Here's how the part is built. I have some questions about the finished solid (model axes, mm). A direction names the side the tool comes from. Coordinates: 2 decimals unless noted, no trailing zeros. Write each loop counter-clockwise with the first axis right and the second up, starting at its lowest first coordinate (ties: lowest second). Pieces come first, ordered by that corner, then holes.
(1) Which directions (+Z, -Z, +X, -X, +Y, -Y) give clear straight access to the entire face, cutting with the end or side of a thin tool? Please do faces 4 (the flat face through (-1, 106, 50)), 5 (the flat face through (-1, 85, 53)), 6 (the flat face through (-1, 86, -55)).
(2) Please list where these lines run through material, in increasing order: probe 1 along X at (y, z) = (111, 12); probe 2 along Z at (x, y) = (2, 154); probe 3 along Y at (x, z) = (-9, -48).
(3) Imagine slicing it at C-C, the plane z = -33.5. List the corners of the cut face in (x, y) for me, plus the area to 4 significant figures.
(4) For pin 1 Ø8 at (x, y) = (-37.5, 79) entering from +Z, with a flat end and sliding along its axis, tell me the tip position at first contact or that it passes through.
(5) Thinking about a two-plate mould opening in Y: for faces 1 (the flat face through (-1, 5, 53)), 2 (the flat face through (-1, 86, -50)), 3 (the flat face through (-1, 0, 1)), which applies, released by +Y, released by -Y, zero draft, split by the parting line, or undercut?
(6) Imagine slicing it at B-B, the plane y = 93. List the corners of the cut face in (x, z) for me.
(7) Imagine slicing it at A-A, the plane x = -57. List the corners of the cut face in (y, z) for me.
```python
from build123d import *

# Parameters (mm, degrees)
SKETCH1_W           = 185
SKETCH1_H           = 110
SKETCH1_W_2         = 175
SKETCH1_H_2         = 100
EXTRUDE_THIN1_DEPTH = 175
SKETCH2_W           = 185
SKETCH2_H           = 110
BOSS_EXTRUDE2_DEPTH = 5
CUT_EXTRUDE2_REACH  = 228.454
SKETCH5_W           = 130
SKETCH5_H           = 80
SKETCH6_R           = 1.5
BOSS_EXTRUDE3_DEPTH = 2


with BuildPart() as part:
    # Sketch1 → Extrude-Thin1 (new body)
    with BuildSketch(Plane(origin=(0, 0, 0), x_dir=(1, 0, 0), z_dir=(0, 1, 0))):
        Rectangle(SKETCH1_W, SKETCH1_H)
        Rectangle(SKETCH1_W_2, SKETCH1_H_2, mode=Mode.SUBTRACT)
    extrude(amount=EXTRUDE_THIN1_DEPTH)

    # Sketch2 → Boss-Extrude2 (add)
    with BuildSketch(Plane.XZ):
        Rectangle(SKETCH2_W, SKETCH2_H)
    extrude(amount=BOSS_EXTRUDE2_DEPTH)

    # Sketch5 → Cut-Extrude2 (cut, up to next)
    with BuildSketch(Plane.XY.offset(55), mode=Mode.PRIVATE) as cut_extrude2_sk1:
        with Locations((0, 45)):
            Rectangle(SKETCH5_W, SKETCH5_H)
    cut_extrude2_tool1 = extrude(cut_extrude2_sk1.sketch, amount=-CUT_EXTRUDE2_REACH, mode=Mode.PRIVATE) & part.part
    add(cut_extrude2_tool1.solids().sort_by_distance((0, 45, 55))[0], mode=Mode.SUBTRACT)

    # Sketch6 → Boss-Extrude3 (add)
    with BuildSketch(Plane.ZY.offset(-65)):
        with Locations(Location((52.5, 7.5, 0), (0, 0, 270))):
            Circle(SKETCH6_R)
    extrude(amount=BOSS_EXTRUDE3_DEPTH)


solid = part.part
```
Recorded:
1. face 4: +Y
1. face 5: +Z
1. face 6: -Z, +X, -X, +Y, -Y
2. probe 1: x = -92.5 to -87.5, 87.5 to 92.5
2. probe 2: z = -55 to -50, 50 to 55
2. probe 3: y = -5 to 0
3. outline: (-92.5, -5) - (92.5, -5) - (92.5, 175) - (87.5, 175) - (87.5, 0) - (-87.5, 0) - (-87.5, 175) - (-92.5, 175) - close
3. area: 2,675 mm2
4. pin 1: stops at z = -50
5. face 1: undercut
5. face 2: zero draft
5. face 3: released by +Y
6. outline: (-92.5, -55) - (92.5, -55) - (92.5, 55) - (-92.5, 55) - close; hole (-87.5, -50) - (87.5, -50) - (87.5, 50) - (-87.5, 50) - close
7. outline: (-5, -55) - (175, -55) - (175, -50) - (0, -50) - (0, 50) - (5, 50) - (5, 55) - (-5, 55) - close; (85, 50) - (175, 50) - (175, 55) - (85, 55) - close
